Verification items for this drawing (mm, ordinates from the low corner). Coordinates: 2 decimals unless noted, no trailing zeros. Order: outer loops, then holes, each group sorted by start corner. A loop starts at its lowest first (then second) coordinate and runs counter-clockwise, first axis right, second up. Notation, with made-up numbers: (69, -10) -> (100, -10) arc R9 cw to (100, 7) -> close; hole circle Ø8 at (60, 25). An arc over 180 degrees is marked (long way). Write item = value, one per line. Start each with the question number.
1. Thickness scan on line 1 along Y through (x, z) = (119.5, 0.6); line 2 along X through (y, z) = (118, 2.2); line 3 along X through (y, z) = (129.5, 0.7) (1 decimal). Record the ranges inside material, lowest first. Write a range as from..to.
2. Cross-section at C-C on z = 1.3. Give the number of separate pieces and of enclosed holes in the cut face.
3. Cross-section at A-A on y = 147. Record the cut outline in (x, z) (1 decimal).
4. Cross-section at D-D on x = 29.5. Record the cut outline in (y, z) (1 decimal).
5. Go/stop test with flat-tipped pins: P1, Ø1, axis at x = 25, z = 2, coming from the +Y side; P2, Ø1.6, axis at y = 74, z = 1, coming from the +X side; P3, Ø1.6, axis at y = 53.5, z = 1.5, coming from the -X side; P4, Ø6, axis at x = 13, y = 45, coming from the -Z side. Record where each tip stops, or that it passes through.
6. Cross-section at B-B on y = 92. Record the cut outline in (x, z) (1 decimal).
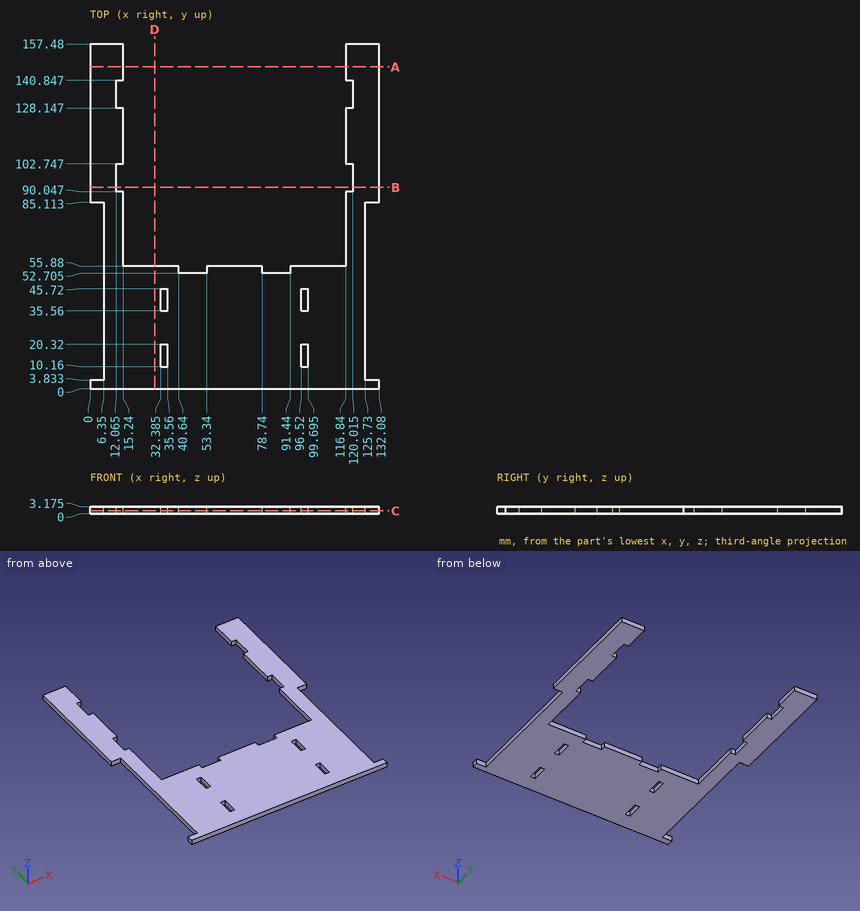
Worked out:
q1.line_1 = 0..90.05, 102.75..128.15, 140.85..157.48
q1.line_2 = 0..15.24, 116.84..132.08
q1.line_3 = 0..12.1, 120..132.1
q2.separate_pieces = 1
q2.enclosed_holes = 4
q3.outline = (0, 0) -> (15.2, 0) -> (15.2, 3.2) -> (0, 3.2) -> close; (116.8, 0) -> (132.1, 0) -> (132.1, 3.2) -> (116.8, 3.2) -> close
q4.outline = (0, 0) -> (55.9, 0) -> (55.9, 3.2) -> (0, 3.2) -> close
q5.P1 = 55.88
q5.P2 = 125.73
q5.P3 = 6.35
q5.P4 = 0
q6.outline = (0, 0) -> (12.1, 0) -> (12.1, 3.2) -> (0, 3.2) -> close; (120, 0) -> (132.1, 0) -> (132.1, 3.2) -> (120, 3.2) -> close
